Autodesk Fusion 360 part; units mm, degrees
sketch "Sketch2" plane through (0, 0, 0) normal (0, 1, 0) x (1, 0, 0)
  arc A0 (0, 0) -> (55, 0) centre (27.5, 15.8771) ccw
  line L0 (0, 0) -> (27.5, 15.8771) construction
  line L1 (27.5, 15.8771) -> (55, 0) construction
  arc A1 (-2.5981, -1.5) -> (57.5981, -1.5) centre (27.5, 15.8771) ccw
  line L2 (0, 0) -> (-2.5981, -1.5)
  line L3 (57.5981, -1.5) -> (55, 0)
  line L4 (27.5, 15.8771) -> (27.5, -52.8095) construction
  line L5 (27.5, 15.8771) -> (10.1229, -14.2209) construction
  line L6 (27.5, 15.8771) -> (44.8771, -14.2209) construction
  line L7 (10.1229, -18.8771) -> (44.8771, -18.8771)
  line L8 (44.8771, -14.2209) -> (44.8771, -18.8771)
  line L9 (10.1229, -14.2209) -> (10.1229, -18.8771)
  line L10 (20.1229, -18.8771) -> (20.1229, -58.8771)
  line L11 (20.1229, -58.8771) -> (35.1229, -58.8771)
  line L12 (35.1229, -58.8771) -> (35.1229, -18.8771)
  dimension "d2" = 55
  dimension "d3" = 120
  dimension "d4" = 3
  dimension "d7" = 30
  dimension "d24" = 30
  dimension "d25" = 40
  dimension "d26" = 10
  dimension "d27" = 15
extrude "Extrude4" add sketch "Sketch2" along normal blind 40 contours A0 A1 L2 L3 | A1 L7 L9 | A1 L7 L8
extrude "Extrude5" add sketch "Sketch2" along normal blind 3 contours L7 L10 L11 L12
fillet "Fillet1" radius 1 7 edges at (10.1229, 20, 14.2209) (10.1229, 20, 18.8771) (44.8771, 20, 18.8771) (44.8771, 20, 14.2209) (27.6229, 3, 18.8771) (35.1229, 1.5, 18.8771) (20.1229, 1.5, 18.8771)
fillet "Fillet2" radius 1 4 edges at (57.5981, 20, 1.5) (55, 20, 0) (-2.5981, 20, 1.5) (0, 20, 0)
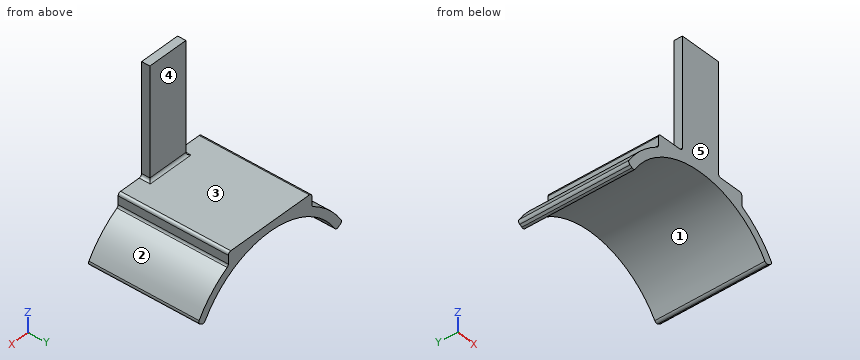
Verification items for the finished model (mm, model axes). Face numbers are marked on the shaded views. A direction names the side the tool comes from. Give positions to 0.01 mm unless a question says otherwise; leave off trailing zeros. Loops run counter-clockwise (first coordinate to the right, second up) from the corner with the lowest first, then second, coordinate; pieces in that order, holes last. Notation, with made-up numbers: M -34.75,-17 L 11.25,-17 A11 cw 11.25,1 Z; hole C -27.75,82 d4. An arc over 180 degrees is marked long. Return JSON: item names as keys, results as strings.
1) Section check D-D, the plane z = 43. Enter the section's corners in (x, y), and give its area (3 significant figures).
Findings:
{"outline": "M 20.12,0 L 35.12,0 L 35.12,3 L 20.12,3 Z", "area": "45.0 mm2"}
2) Section check B-B, the plane y = 18. Enter the section's corners in (x, z).
Findings:
{"outline": "M -2.07,2.38 A1 ccw -1.72,0.99 L -0.85,0.49 A1 ccw 0.5,0.83 A31.75 cw 54.5,0.83 A1 ccw 55.85,0.49 L 56.72,0.99 A1 ccw 57.07,2.38 A34.75 ccw 45.36,13.94 A1 cw 44.88,14.79 L 44.88,17.88 A1 ccw 43.88,18.88 L 11.12,18.88 A1 ccw 10.12,17.88 L 10.12,14.79 A1 cw 9.64,13.94 A34.75 ccw Z"}
3) Section check C-C, the plane x = 33. Enter the section's corners in (y, z).
Findings:
{"outline": "M 0,15.4 L 40,15.4 L 40,18.88 L 4,18.88 A1 cw 3,19.88 L 3,58.88 L 0,58.88 Z"}
4) Tool access check on the marked faces 4 and 5. Record the directions out of +Z, -Z, +X, -X, +Y, -Y that give a thin tool (end or side, any length) a straight path to the whole face; none if there is none.
Findings:
{"face 4": "+Z, +X, -X, +Y", "face 5": "+Z, -Z, +X, -X, -Y"}
5) Gauge pin test, flat ends, axial feed: P1, Ø4.5, axis at x = 27.5, z = 39.5, coming from the +Y side; P2, Ø3, axis at x = 39, y = 24.5, coming from the +Z side; P3, Ø1.5, axis at y = 21, z = 20, coming from the +X side; P4, Ø3.5, axis at y = 1, z = 33, coming from the -X side. Record the tip position at first contact, or that the pin passes through.
Findings:
{"P1": "stops at y = 3", "P2": "stops at z = 18.88", "P3": "passes through", "P4": "stops at x = 20.12"}
6) Mould release check, pull along X, two halves, no side actions. Record for the marked faces 1, 2 and 3: released by +X, released by -X, zero draft, split by the parting line, or undercut.
Findings:
{"face 1": "undercut", "face 2": "released by +X", "face 3": "zero draft"}
7) Section check A-A, the plane z = 8.5. Enter the section's corners in (x, y).
Findings:
{"outline": "M 2.73,0 L 7.15,0 L 7.15,40 L 2.73,40 Z; M 47.85,0 L 52.27,0 L 52.27,40 L 47.85,40 Z"}
8) Material ranges on L1, parallel to X at y = 16, z = 16.5; L2, parallel to X at y = 31.5, z = 13.5; L3, parallel to X at y = 23, z = 5.5, recorded low to high. Write a range as [from, to].
Findings:
{"L1": "x = [10.12, 44.88]", "L2": "x = [8.93, 15.45], [39.55, 46.07]", "L3": "x = [0.1, 4.02], [50.98, 54.9]"}
